Read the model definition and answer for the solid it produces. Units are mm, in the model's axes. Face numbers are marked on the shaded views. Round coordinates to 2 decimals unless told otherwise and drop trailing zeros. Return JSON: item names as keys, results as strings. Group by question number.
(1) Given pin 1 (1.2 mm diameter, centred on y = 24, z = 47.5, fed in from +X); pin 2 (1 mm diameter, centred on x = -26.5, z = 45, fed in from -Y); pin 3 (12 mm diameter, centred on x = 10.5, z = 35.5, fed in from +Y); pin 4 (1 mm diameter, centred on x = 7.5, z = 20, fed in from +Y), each flat-ended and moving along its own axis, determine where each tip first touches the part or whether it passes through.
(2) The mould has two halves that part along X. Classify the marked faces 1 and 2: released by +X, released by -X, zero draft, split by the parting line, or undercut.
(3) A cutting plane is placed at A-A on y = 14.5. State how many separate pieces and enclosed holes the cut face has, then the cut area to 3 significant figures.
(4) Straight lines are drawn through the part: line 1 (X direction, y = 24, z = 58); line 2 (Y direction, x = -18.5, z = 53). For each, find the intervals that lie inside material, in ascending order.
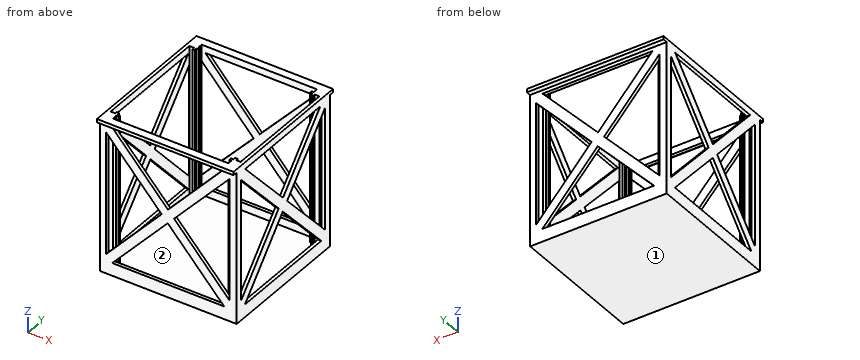
```python
from build123d import *

# Parameters (mm, degrees)
F1_DEPTH  = 64
F4_DEPTH  = 1.4
F6_DEPTH  = 2
F8_COUNT  = 4
F9_W      = 58
F9_H      = 1.4429360032
F10_DEPTH = 2


with BuildPart() as f1:
    # F0 (on Top) → F1 (new body)
    with BuildSketch(Plane.XY):
        Polygon((0, -27.6), (0, -29), (29, -29), (24.6101661921, -24.6101661921), (23.5489513725, -24.6101661921), (23.5489513725, -25.6), (24.5, -25.6), (24.5, -27.6), align=None)
    extrude(amount=F1_DEPTH)

    # F2: F1 across plane


with BuildPart() as f1_1:
    add(f1.part)
    add(f1.part.mirror(Plane.YZ))

    # F3 (on face) → F4 (cut)
    with BuildSketch(Plane.XZ.offset(29)):
        Polygon((-2.8809057808, 32.3860045068), (-26.4172293246, 58.0803863704), (-26.4172293246, 6.2722163275), align=None)
        Polygon((22.9713302106, 61.0693208873), (-23.7129572779, 61.0693208873), (-0.1818502389, 35.3806338326), align=None)
        Polygon((25.9602628648, 58.6964643958), (2.4026971831, 32.5591078504), (25.9602628648, 6.8415361457), align=None)
        Polygon((23.6471185492, 3.425611183), (-0.2963583588, 29.5644785245), (-23.855285719, 3.425611183), align=None)
    extrude(amount=-F4_DEPTH, mode=Mode.SUBTRACT)

    # F5 (on face) → F6 (join)
    with BuildSketch(Plane(origin=(0, 0, 0), x_dir=(1, 0, 0), z_dir=(0, 0, -1))):
        Polygon((29, 29), (-29, 29), (0, 0), align=None)
    extrude(amount=F6_DEPTH)


with BuildPart() as f8_1:
    # F8: instance of F1
    add(f1_1.part.rotate(Axis((0, 0, 25.6520500407), (0, 0, -1)), 1 * 360 / F8_COUNT))


with BuildPart() as f8_2:
    # F8: instance of F1
    add(f1_1.part.rotate(Axis((0, 0, 25.6520500407), (0, 0, -1)), 2 * 360 / F8_COUNT))


with BuildPart() as f8_3:
    # F8: instance of F1
    add(f1_1.part.rotate(Axis((0, 0, 25.6520500407), (0, 0, -1)), 3 * 360 / F8_COUNT))


with BuildPart() as f10:
    # F9 (on face) → F10 (new body)
    with BuildSketch(Plane.XZ.offset(29)):
        with Locations((0, 63.2785319984)):
            Rectangle(F9_W, F9_H)
    extrude(amount=F10_DEPTH)


with BuildPart() as f1_2:
    add(f1_1.part)

    add(f8_1.part)  # F11 merges F8_1

    add(f8_2.part)  # F11 merges F8_2

    add(f8_3.part)  # F11 merges F8_3

    add(f10.part)  # F11 merges F10
    # F11: F10 across plane
    add(f10.part.mirror(Plane.XZ))


solid = f1_2.part
```
Checks:
{
 "1": {"pin 1": "stops at x = 27.6", "pin 2": "stops at y = -29", "pin 3": "stops at y = 29", "pin 4": "passes through"},
 "2": {"face 1": "zero draft", "face 2": "undercut"},
 "3": {"separate pieces": "7", "enclosed holes": "0", "area": "166 mm^2"},
 "4": {"line 1": "x = -29 to -27.6, -25.6 to -24.61, 24.61 to 25.6, 27.6 to 29", "line 2": "y = -29 to -27.6, 27.6 to 29"}
}
